Part model, mm, in its own coordinate system. A direction names the side the tool comes from. Round coordinates to 2 decimals unless told otherwise and drop trailing zeros. Loops run counter-clockwise (first coordinate to the right, second up) from the corner with the lowest first, then second, coordinate; pieces in that order, holes last. Notation, with made-up numbers: M 63,58 L 106,58 A11 ccw 106,67 Z; hole C 58.25,1.25 d3. An arc over 180 degrees is marked long. Put each result on its own line as item: value. Start each with the question number.
1) Slice it at C-C on x = 76. Give the cut face in (y, z).
2) Drop flat-ended pins along their axis: pin 1 Ø5 at (x, z) = (57.5, 0) entering from -Y; pin 2 Ø10.5 at (y, z) = (19.5, -21.5) entering from +X; pin 3 Ø5 at (x, z) = (37, -18.5) entering from -Y; pin 4 Ø7.5 at (x, y) = (90.5, -2) entering from -Z. Give the stop position or say it passes through.
3) Pull direction Y, two halves, no side cores. Call faces 5 (the flat face through (12.27, -30.5, -36.33)), 6 (the flat face through (17.535, -41.678, -50.364)), 7 (the cylindrical face through (68.84, -0.1, -38.23)), 8 (the flat face through (17.535, 23.644, -60.776)): +Y half, -Y half, draft (parallel to the pull), parting line (faces both ways), or undercut.
4) Probe line 1 along Z through (x, y) = (30, 9.5); line 2 along Y through (x, z) = (67, 0.5); line 3 along Z through (x, y) = (76, 3.5). List the from-to ranges inside material, lowest first.
5) Slice it at B-B on z = -17. Give the cut face in (x, y), then the cut area to 3 significant figures.
6) Slice it at A-A on x = 50. Give the cut face in (y, z).
7) Slice it at D-D on z = 0. State how many separate pieces and enclosed holes the cut face has, then the cut area to 3 significant figures.
8) Which spindle directions (+Z, -Z, +X, -X, +Y, -Y) get a long thin tool onto all of the face, cutting with end or side? Do faces 1 (the flat face through (33, 0, -37.874)), 2 (the cylindrical face through (59, -10, 0)), 3 (the flat face through (20, -15, -46)), 4 (the flat face through (49, 5, -7.75)). Say none if no direction does.
```python
from build123d import *

# Parameters (mm, degrees)
F0_W         = 15
F0_H         = 15
F1_DEPTH     = 20
F3_DEPTH     = 15
F4_R         = 1.5
F5_DEPTH     = 5.5
F6_R         = 1.5
F7_DEPTH     = 5.5
F8_W         = 15
F8_H         = 15
F9_DEPTH     = 47.5
F10_R        = 4
F11_DEPTH    = 19.374355653
F13_DEPTH    = 47.5
F14_R        = 2.75
F15_DEPTH    = 52.6205461814
F16_DEPTH    = 20
F17_W        = 67.5
F17_H        = 14.8660254038
F17_R        = 4
F18_DEPTH    = 11
F19_W        = 14.8660254038
F19_H        = 26.3910161514
F20_DEPTH    = 67.501
F21_SIZE     = 5
F22_R        = 1.5
F23_DEPTH    = 58.6875334795
F24_W        = 15.5
F24_H        = 15.5
F25_DEPTH    = 67.501
F26_W        = 15.5
F26_H        = 15.5
F27_DEPTH    = 51.2593302492
F28_W        = 15.5
F28_H        = 15.5
F29_DEPTH    = 51.2593302492
F30_DEPTH    = 32
F31_R        = 2.75
F32_DEPTH    = 52.6205461814
F33_R        = 8
F33_R_2      = 2.75
F34_DEPTH    = 14.8660254038
F36_DEPTH    = 99.5
F37_W        = 27
F37_H        = 4.75
F38_DEPTH    = 99.501
F39_T1_DEPTH = 40.5828552834
F39_T3_DEPTH = 31.4668298797
F39_T5_DEPTH = 31.4668298797
F40_R        = 5
F41_SIZE     = 2


# Not quite as in the source:
# - a fillet or chamfer that OpenCascade refuses, or shapes differently, is made with other operations: its cross-section is extruded or revolved along the edge and cut away or added
# - an extrude ends at something that could not be found from the text; its depth is read off the source's solid


with BuildPart() as f1:
    # F0 (on Right) → F1 (new body)
    with BuildSketch(Plane.YZ):
        Polygon((45.1865334795, -51.2653718044), (8.3715789032, 12.5), (-8.3715789032, 12.5), (-45.1865334795, -51.2653718044), (-22.6698729811, -64.2653718044), (0, -25), (22.6698729811, -64.2653718044), align=None)
        Rectangle(F0_W, F0_H, mode=Mode.SUBTRACT)
    extrude(amount=F1_DEPTH)

    # F2 (on face) → F3 (cut)
    with BuildSketch(Plane.YZ.offset(20)):
        Polygon((-20.4233937587, -19.374355653), (-40.4233937587, -54.0153718044), (-27.4330127019, -61.5153718044), (-7.4330127019, -26.874355653), align=None)
        Polygon((27.4330127019, -61.5153718044), (40.4233937587, -54.0153718044), (20.4233937587, -19.374355653), (7.4330127019, -26.874355653), align=None)
    extrude(amount=-F3_DEPTH, mode=Mode.SUBTRACT)

    # F4 (on face) → F5 (cut, through all)
    with BuildSketch(Plane(origin=(0, -11.6913429511, 6.75), x_dir=(1, 0, 0), z_dir=(0, -0.8660254038, 0.5))):
        with Locations((12.5, -36.9903810568)):
            Circle(F4_R)
        with Locations((12.5, -56.9903810568)):
            Circle(F4_R)
    extrude(amount=-F5_DEPTH, mode=Mode.SUBTRACT)

    # F6 (on face) → F7 (cut, through all)
    with BuildSketch(Plane(origin=(0, 11.6913429511, 6.75), x_dir=(-1, 0, 0), z_dir=(0, 0.8660254038, 0.5))):
        with Locations((-12.5, -56.9903810568)):
            Circle(F6_R)
        with Locations((-12.5, -36.9903810568)):
            Circle(F6_R)
    extrude(amount=-F7_DEPTH, mode=Mode.SUBTRACT)

    # F8 (on face) → F9 (join)
    with BuildSketch(Plane.YZ.offset(20)):
        Polygon((8.3715789032, 12.5), (-8.3715789032, 12.5), (-13.5, 3.6173140978), (-13.5, -23.3715789032), (-7.4330127019, -26.874355653), (7.4330127019, -26.874355653), (13.5, -23.3715789032), (13.5, 3.6173140978), align=None)
        Rectangle(F8_W, F8_H, mode=Mode.SUBTRACT)
    extrude(amount=F9_DEPTH)

    # F10 (on face) → F11 (cut, through all)
    with BuildSketch(Plane(origin=(0, 0, -26.874355653), x_dir=(1, 0, 0), z_dir=(0, 0, -1))):
        with Locations((50, 0)):
            Circle(F10_R)
    extrude(amount=-F11_DEPTH, mode=Mode.SUBTRACT)

    # F12 (on face) → F13 (cut, through all)
    with BuildSketch(Plane.YZ.offset(67.5)):
        Polygon((-13.5, -23.3715789032), (-7.4330127019, -26.874355653), (-7.4330127019, -10.25), (-13.5, -10.25), align=None)
        Polygon((7.4330127019, -10.25), (7.4330127019, -26.874355653), (13.5, -23.3715789032), (13.5, -10.25), align=None)
    extrude(amount=-F13_DEPTH, mode=Mode.SUBTRACT)

    # F14 (on face) → F15 (cut, through all)
    with BuildSketch(Plane.XZ.offset(7.4330127019)):
        with Locations((36.9997965198, -18.5)):
            Circle(F14_R)
    extrude(amount=-F15_DEPTH, mode=Mode.SUBTRACT)

    # F16 (add, through all): a face of the model
    f16_faces = [f1.faces().sort_by_distance(p)[0] for p in [
        (20, 0, -26.2495704353),
    ]]
    extrude(f16_faces, amount=F16_DEPTH)

    # F17 (on face) → F18 (join, through all)
    with BuildSketch(Plane(origin=(0, 0, -26.874355653), x_dir=(1, 0, 0), z_dir=(0, 0, -1))):
        with Locations((33.75, 0)):
            Rectangle(F17_W, F17_H)
        with Locations((50, 0)):
            Circle(F17_R, mode=Mode.SUBTRACT)
    extrude(amount=F18_DEPTH)

    # F19 (on face) → F20 (cut, through all)
    with BuildSketch(Plane(origin=(0, 0, 0), x_dir=(0, -1, 0), z_dir=(-1, 0, 0))):
        with Locations((0, -51.0698637287)):
            Rectangle(F19_W, F19_H)
    extrude(amount=-F20_DEPTH, mode=Mode.SUBTRACT)

    # F21
    f21_edges = [f1.edges().sort_by_distance(p)[0] for p in [
        (20, -42.804964, -52.640372),
        (20, -25.051443, -62.890372),
        (20, 25.051443, -62.890372),
        (20, 42.804964, -52.640372),
    ]]
    chamfer(f21_edges, length=F21_SIZE)

    # F22 (on face) → F23 (cut, through all)
    with BuildSketch(Plane.XZ.offset(13.5)):
        with Locations((30, 0)):
            Circle(F22_R)
        with Locations((57.5, 0)):
            Circle(F22_R)
    extrude(amount=-F23_DEPTH, mode=Mode.SUBTRACT)

    # F24 (on face) → F25 (cut, through all)
    with BuildSketch(Plane(origin=(0, 0, 0), x_dir=(0, -1, 0), z_dir=(-1, 0, 0))):
        Rectangle(F24_W, F24_H)
    extrude(amount=-F25_DEPTH, mode=Mode.SUBTRACT)

    # F26 (on face) → F27 (cut, through all)
    with BuildSketch(Plane(origin=(0, -13.4951905284, -23.374355653), x_dir=(1, 0, 0), z_dir=(0, -0.5, -0.8660254038))):
        with Locations((12.5, 0.5)):
            Rectangle(F26_W, F26_H)
    extrude(amount=F27_DEPTH, mode=Mode.SUBTRACT)

    # F28 (on face) → F29 (cut, through all)
    with BuildSketch(Plane(origin=(0, 13.4951905284, -23.374355653), x_dir=(1, 0, 0), z_dir=(0, 0.5, -0.8660254038))):
        with Locations((12.5, -0.5)):
            Rectangle(F28_W, F28_H)
    extrude(amount=F29_DEPTH, mode=Mode.SUBTRACT)

    # F30 (add): a face of the model
    f30_faces = [f1.faces().sort_by_distance(p)[0] for p in [
        (67.5, 0, -13.0224065519),
    ]]
    extrude(f30_faces, amount=F30_DEPTH)

    # F31 (on face) → F32 (cut, through all)
    with BuildSketch(Plane.XZ.offset(7.4330127019)):
        with Locations((91, -18.5)):
            Circle(F31_R)
        with Locations((76, -33.5)):
            Circle(F31_R)
    extrude(amount=-F32_DEPTH, mode=Mode.SUBTRACT)

    # F33 (on face) → F34 (join, through all)
    with BuildSketch(Plane.XZ.offset(7.4330127019)):
        with Locations((76, -33.5)):
            Circle(F33_R)
        with Locations((76, -33.5)):
            Circle(F33_R_2, mode=Mode.SUBTRACT)
    extrude(amount=-F34_DEPTH)

    # F35 (on face) → F36 (join, through all)
    with BuildSketch(Plane.YZ.offset(99.5)):
        Polygon((-13.5, 3.6173140978), (-8.3715789032, 12.5), (-13.5, 12.5), align=None)
        Polygon((13.5, 12.5), (8.3715789032, 12.5), (13.5, 3.6173140978), align=None)
    extrude(amount=-F36_DEPTH)

    # F37 (on face) → F38 (cut, through all)
    with BuildSketch(Plane.YZ.offset(99.5)):
        with Locations((0, 10.125)):
            Rectangle(F37_W, F37_H)
    extrude(amount=-F38_DEPTH, mode=Mode.SUBTRACT)

    # F39: chamfer of 5 on 5 edges, made by hand

    # F39_s2 → F39_t1 (cut)
    with BuildSketch(Plane.XZ.offset(-20.2914276417)):
        Polygon((99.5, -32.874355653), (94.5, -37.874355653), (99.5, -37.874355653), align=None)
    extrude(amount=F39_T1_DEPTH, mode=Mode.SUBTRACT)

    # F39_s4 → F39_t3 (cut)
    with BuildSketch(Plane.XZ.offset(-5.1084149398)):
        Polygon((94.5, 7.75), (99.5, 2.75), (99.5, 7.75), align=None)
    extrude(amount=F39_T3_DEPTH, mode=Mode.SUBTRACT)

    # F39_s6 → F39_t5 (cut)
    with BuildSketch(Plane.XZ.offset(-26.3584149398)):
        Polygon((94.5, 7.75), (99.5, 2.75), (99.5, 7.75), align=None)
    extrude(amount=F39_T5_DEPTH, mode=Mode.SUBTRACT)

    # F40
    f40_edges = [f1.edges().sort_by_distance(p)[0] for p in [
        (69.301865, 0, -37.874356),
        (82.698135, 0, -37.874356),
    ]]
    fillet(f40_edges, radius=F40_R)

    # F41
    f41_edges = [f1.edges().sort_by_distance(p)[0] for p in [
        (28.5, -13.5, 0),
        (56, -13.5, 0),
        (11, -30.186533, -25.28461),
        (11, -40.186533, -42.605118),
        (56, 13.5, 0),
        (28.5, 13.5, 0),
        (14, 30.186533, -25.28461),
        (14, 40.186533, -42.605118),
    ]]
    chamfer(f41_edges, length=F41_SIZE)


solid = f1.part
```
Recorded:
1. outline: M -13.5,-10.25 L -7.43,-10.25 L -7.43,-30.75 L 7.43,-30.75 L 7.43,-10.25 L 13.5,-10.25 L 13.5,7.75 L 7.75,7.75 L 7.75,-7.75 L -7.75,-7.75 L -7.75,7.75 L -13.5,7.75 Z; M -7.43,-41.5 L 7.43,-41.5 L 7.43,-36.25 L -7.43,-36.25 Z
2. pin 1: stops at y = -12.5
2. pin 2: stops at x = 20
2. pin 3: passes through
2. pin 4: stops at z = -37.87
3. face 5: undercut
3. face 6: -Y half
3. face 7: draft
3. face 8: +Y half
4. line 1: z = -10.25 to -1.5, 1.5 to 7.75
4. line 2: y = -13.5 to -7.75, 7.75 to 13.5
4. line 3: z = -41.5 to -36.25, -30.75 to -7.75
5. outline: M 0,-25.4 L 20,-25.4 L 20,-7.43 L 34.69,-7.43 L 34.69,7.43 L 20,7.43 L 20,25.4 L 0,25.4 Z; M 39.3,-7.43 L 88.7,-7.43 L 88.7,7.43 L 39.3,7.43 Z; M 93.3,-7.43 L 99.5,-7.43 L 99.5,7.43 L 93.3,7.43 Z; hole C 50,0 d8
5. area: 2,010 mm2
6. outline: M -13.5,-10.25 L -7.43,-10.25 L -7.43,-37.87 L -4,-37.87 L -4,-7.75 L -7.75,-7.75 L -7.75,7.75 L -13.5,7.75 Z; M 4,-37.87 L 7.43,-37.87 L 7.43,-10.25 L 13.5,-10.25 L 13.5,7.75 L 7.75,7.75 L 7.75,-7.75 L 4,-7.75 Z
7. separate pieces: 6
7. enclosed holes: 0
7. area: 1,140 mm2
8. face 1: -Z, -X
8. face 2: +Y, -Y
8. face 3: -Z, +X, -Y
8. face 4: +Z, +X, -X
